Input: part model. Units: mm. Frame: model coordinates. A direction names the side the tool comes from. Round coordinates to 2 decimals unless told otherwise and drop trailing zeros. Loops run counter-clockwise (first coordinate to the right, second up) from the corner with the lowest first, then second, coordinate; pieces in that order, holes last.
1) Ray query, line 1 along X through (y, z) = (31.5, 1.5); line 2 along Z through (x, y) = (-1, 76). Return the intervals inside material, ascending.
2) Section A-A, the plane y = 20. Return loops of the section in (x, z), and give its area (3 significant figures).
3) First-contact query: pin 1 (8 mm diameter, centred on x = 0.5, z = -6, fed in from +Y); pin 2 (4 mm diameter, centred on x = 0, z = -3.5, fed in from -Y); pin 3 (6 mm diameter, centred on y = 63, z = -5.5, fed in from +X). Flat tips, straight axial feed; report the tip coordinate or a pass-through.
4) Access query for faces 1 (the face through (13.05, 20, 0)), 2 (the face through (-11.57, 17.9, -0.47)), 3 (the face through (0, 20, -10.05)). Directions: +Z, -Z, +X, -X, +Y, -Y. A direction counts if a zero-diameter tool reaches every point of the face in a straight line with its end or side. Return the directions, or none.
5) Draft query along Z for faces 4 (the face through (0, 20, -13.05)), 5 (the face through (0, 20, 13.05)), 6 (the face through (0, 20, 10.05)), 7 (the face through (12, 0, 0)). Return one class per face: pulls with the +Z half, pulls with the -Z half, needs draft (parallel to the pull), parting line crosses it, or undercut.
Autodesk Inventor part; units mm, degrees
ref_plane "Work Plane1" through (0, 80, 0) normal (0, 1, 0) x (1, 0, 0)
ref_plane "YZ Plane" through (0, 0, 0) normal (1, 0, 0) x (0, 1, 0)
ref_plane "XZ Plane" through (0, 0, 0) normal (0, 1, 0) x (-1, 0, 0)
sketch "Sketch2" plane through (0, 0, 0) normal (0, 1, 0) x (-1, 0, 0)
  line L0 (10.05, 10.05) -> (-10.05, 10.05)
  line L1 (-10.05, 10.05) -> (-10.05, -10.05)
  line L2 (-10.05, -10.05) -> (10.05, -10.05)
  line L3 (10.05, -10.05) -> (10.05, 10.05)
  line L4 (10.05, 10.05) -> (-10.05, -10.05) construction
  line L5 (-10.05, 10.05) -> (10.05, -10.05) construction
  line L6 (13.05, 13.05) -> (-13.05, 13.05)
  line L7 (-13.05, 13.05) -> (-13.05, -13.05)
  line L8 (-13.05, -13.05) -> (13.05, -13.05)
  line L9 (13.05, -13.05) -> (13.05, 13.05)
  point P0 (0, 0)
  dimension "d19" = 20.1
  dimension "d20" = 3
extrude "Extrusion2" add sketch "Sketch2" along normal blind 40
ref_plane "Work Plane1" through (0, 80, 0) normal (0, 1, 0) x (1, 0, 0)
sketch "Sketch3" plane through (0, 80, 0) normal (0, 1, 0) x (1, 0, 0)
  line L0 (-10.05, -10.05) -> (-10.05, 10.05)
  line L1 (10.05, 10.05) -> (10.05, -10.05)
  line L2 (-10.05, -10.05) -> (10.05, 10.05) construction
  circle A0 centre (0, 0) radius 5
  dimension "d24" = 10
sketch "Sketch4" plane through (0, 40, 0) normal (0, 1, 0) x (1, 0, 0)
  line L0 (13.05, -13.05) -> (13.05, 13.05)
  line L1 (13.05, 13.05) -> (-13.05, 13.05)
  line L2 (-13.05, 13.05) -> (-13.05, -13.05)
  line L3 (-13.05, -13.05) -> (13.05, -13.05)
  line L4 (-10.05, -10.05) -> (-10.05, 10.05) construction
  line L5 (-10.05, 10.05) -> (10.05, 10.05)
  line L6 (10.05, 10.05) -> (10.05, -10.05)
  line L7 (10.05, -10.05) -> (-10.05, -10.05)
  point P0 (0, 0)
loft "Loft1" add profiles "Sketch3", "Sketch4"
sketch "Sketch5" plane through (0, 80, 0) normal (0, 1, 0) x (1, 0, 0)
  arc A0 (-3.5355, 3.5355) -> (-3.5355, -3.5355) centre (0, 0) ccw
  line L0 (-5, 0) -> (5, 0)
  arc A1 (3.5355, -3.5355) -> (3.5355, 3.5355) centre (0, 0) ccw
  arc A2 (-3.5355, -3.5355) -> (3.5355, -3.5355) centre (0, 0) ccw
  arc A3 (3.5355, -3.5355) -> (3.5355, 3.5355) centre (0, 0) ccw
  arc A4 (3.5355, 3.5355) -> (-3.5355, 3.5355) centre (0, 0) ccw
  arc A5 (-3.5355, 3.5355) -> (-3.5355, -3.5355) centre (0, 0) ccw
  point P0 (-3.5355, -3.5355)
revolve "Revolution1" add sketch "Sketch5" angle 360 about axis through (-5, 80, 0) along (1, 0, 0) contours L0 A1 A2 A0
sketch "Sketch6" plane through (-13.05, 0, -13.05) normal (-1, 0, 0) x (0, 0, 1)
  line L0 (9.5145, 80) -> (0, 40)
  line L1 (26.1, 0) -> (26.1, 40)
  line L2 (0, 40) -> (26.1, 0) construction
  circle A0 centre (13.05, 20) radius 2.15
  point P0 (13.05, 0)
  dimension "d30" = 4.3
extrude "Extrusion3" cut sketch "Sketch6" against normal blind 18.855
equation "\"l1\" = 1"
properties part number "Pies" material "PET Plastic"
Final values:
1. line 1: x = -13.05 to -10.05, 10.05 to 13.05
1. line 2: z = -5.75 to -2.83, 2.83 to 5.75
2. outline: (-13.05, -13.05) - (13.05, -13.05) - (13.05, 13.05) - (-13.05, 13.05) - (-13.05, 2.15) - (-10.05, 2.15) - (-10.05, 10.05) - (10.05, 10.05) - (10.05, -10.05) - (-10.05, -10.05) - (-10.05, -2.15) - (-13.05, -2.15) - close
2. area: 264 mm2
3. pin 1: stops at y = 80
3. pin 2: stops at y = 40
3. pin 3: stops at x = 8.77
4. face 1: +Z, -Z, +X, +Y, -Y
4. face 2: -X
4. face 3: -Y
5. face 4: pulls with the -Z half
5. face 5: pulls with the +Z half
5. face 6: undercut
5. face 7: needs draft
